Build history of the part. All positions in model axes, mm. A direction names the side the tool comes from. Round coordinates to 2 decimals unless told otherwise and drop trailing zeros. Loops run counter-clockwise (first coordinate to the right, second up) from the corner with the lowest first, then second, coordinate; pieces in that order, holes last. Notation, with made-up numbers: (76, -13) - (87, -13) arc R22 ccw to (87, -2) - close; hole circle Ø9 at (45.5, 45). An arc over 180 degrees is marked (long way). Put each result on its own line as item: value. Start each with the question number.
Autodesk Inventor part; units mm, degrees
ref_plane "РабПлоскость1" through (0, 28, 0) normal (0, 1, 0) x (-1, 0, 0)
ref_plane "YZ Plane" through (0, 0, 0) normal (1, 0, 0) x (0, 1, 0)
ref_plane "XY Plane" through (0, 0, 0) normal (0, 0, 1) x (1, 0, 0)
sketch "Эскиз1" plane through (0, 0, 0) normal (0, 1, 0) x (-1, 0, 0)
  line L0 (-2, 80) -> (2, 80)
  line L1 (2, 80) -> (2, -80)
  line L2 (2, -80) -> (-2, -80)
  line L3 (-2, -80) -> (-2, 80)
  line L4 (60, 32) -> (-60, 32)
  line L5 (-60, 32) -> (-60, 36)
  line L6 (-60, 36) -> (60, 36)
  line L7 (60, 36) -> (60, 32)
  line L8 (60, -32) -> (-60, -32)
  line L9 (-60, -32) -> (-60, -36)
  line L10 (-60, -36) -> (60, -36)
  line L11 (60, -36) -> (60, -32)
  line L12 (60, 32) -> (60, -32) construction
  line L13 (2, -80) -> (2, -80)
  line L14 (2, -80) -> (-2, -80)
  point P0 (0, 0)
  point P1 (0, -32)
  point P2 (60, 0)
  point P3 (0, -80)
  point P4 (2, 0)
  dimension "d1" = 120
  dimension "d3" = 4
  dimension "d4" = 4
  dimension "d5" = 4
  dimension "d26" = 32
  dimension "d27" = 32
  dimension "d28" = 80
  dimension "d29" = 80
  dimension "d32" = 44
extrude "Выдавливание1" add sketch "Эскиз1" along normal blind 56
ref_plane "РабПлоскость1" through (0, 28, 0) normal (0, 1, 0) x (-1, 0, 0)
sketch "Эскиз2" plane through (0, 0, 0) normal (0, 1, 0) x (-1, 0, 0)
  line L0 (-2, 36) -> (-2, 80) construction
  line L1 (-2, 80) -> (2, 80) construction
  line L2 (2, 80) -> (2, 36) construction
  line L3 (2, 36) -> (60, 36) construction
  line L4 (60, 36) -> (60, 32) construction
  line L5 (60, 32) -> (2, 32) construction
  line L6 (2, 32) -> (2, -32) construction
  line L7 (60, -32) -> (2, -32) construction
  line L8 (60, -36) -> (60, -32) construction
  line L9 (2, -36) -> (60, -36) construction
  line L10 (2, -36) -> (2, -80) construction
  line L11 (2, -80) -> (-2, -80) construction
  line L12 (-2, -80) -> (-2, -36) construction
  line L13 (-60, -36) -> (-2, -36) construction
  line L14 (-60, -32) -> (-60, -36) construction
  line L15 (-2, -32) -> (-60, -32) construction
  line L16 (-2, -32) -> (-2, 32) construction
  line L17 (-2, 32) -> (-60, 32) construction
  line L18 (-60, 32) -> (-60, 36) construction
  line L19 (-60, 36) -> (-2, 36) construction
  line L20 (-2, 32) -> (-6, 32)
  line L21 (-6, 32) -> (-6, 29)
  line L22 (-5, 28) -> (-2, 28)
  line L23 (-2, 28) -> (-2, 32)
  circle A0 centre (-4, 30) radius 1
  arc A1 (-6, 29) -> (-5, 28) centre (-5, 29) ccw
  line L24 (-2, -36) -> (-6, -36)
  line L25 (-6, -36) -> (-6, -39)
  line L26 (-5, -40) -> (-2, -40)
  line L27 (-2, -40) -> (-2, -36)
  circle A2 centre (-4, -38) radius 1
  arc A3 (-6, -39) -> (-5, -40) centre (-5, -39) ccw
  line L28 (-60, 34) -> (60, 34) construction
  line L29 (-60, -34) -> (60, -34) construction
  line L30 (0, 80) -> (0, -80) construction
  line L31 (-2, 36) -> (-6, 36)
  line L32 (-6, 36) -> (-6, 39)
  line L33 (-5, 40) -> (-2, 40)
  line L34 (-2, 40) -> (-2, 36)
  circle A4 centre (-4, 38) radius 1
  arc A5 (-5, 40) -> (-6, 39) centre (-5, 39) ccw
  line L35 (2, 32) -> (6, 32)
  line L36 (6, 32) -> (6, 29)
  line L37 (5, 28) -> (2, 28)
  line L38 (2, 28) -> (2, 32)
  circle A6 centre (4, 30) radius 1
  arc A7 (5, 28) -> (6, 29) centre (5, 29) ccw
  arc A8 (6, 39) -> (5, 40) centre (5, 39) ccw
  line L39 (5, 40) -> (2, 40)
  line L40 (2, 40) -> (2, 36)
  line L41 (6, 36) -> (6, 39)
  line L42 (2, 36) -> (6, 36)
  circle A9 centre (4, 38) radius 1
  line L43 (-2, -28) -> (-2, -32)
  line L44 (-2, -32) -> (-6, -32)
  circle A10 centre (-4, -30) radius 1
  line L45 (-6, -32) -> (-6, -29)
  arc A11 (-5, -28) -> (-6, -29) centre (-5, -29) ccw
  line L46 (-5, -28) -> (-2, -28)
  line L47 (2, -40) -> (2, -36)
  line L48 (2, -36) -> (6, -36)
  circle A12 centre (4, -38) radius 1
  line L49 (6, -36) -> (6, -39)
  arc A13 (5, -40) -> (6, -39) centre (5, -39) ccw
  line L50 (5, -40) -> (2, -40)
  line L51 (2, -28) -> (2, -32)
  line L52 (2, -32) -> (6, -32)
  line L53 (6, -32) -> (6, -29)
  line L54 (5, -28) -> (2, -28)
  arc A14 (6, -29) -> (5, -28) centre (5, -29) ccw
  circle A15 centre (4, -30) radius 1
  point P0 (0, 0)
  point P1 (-6, 28)
  point P2 (-6, -40)
  point P3 (-6, 40)
  point P4 (6, 28)
  point P5 (6, 40)
  point P6 (-6, -28)
  point P7 (2, -32)
  point P8 (6, -40)
  point P9 (6, -28)
  dimension "d11" = 4
  dimension "d12" = 4
  dimension "d13" = 2
  dimension "d15" = 1
  dimension "d16" = 2
  dimension "d17" = 2
  dimension "d18" = 4
  dimension "d19" = 4
  dimension "d20" = 2
  dimension "d21" = 1
  dimension "d22" = 2
  dimension "d23" = 2
extrude "Выдавливание2" add sketch "Эскиз2" along normal blind 2
mirror "Зеркальное отражение1" about plane through (0, 28, 0) normal (0, 1, 0) of "Выдавливание2"
extrude "Выдавливание3" add sketch "Эскиз1" along normal up to surface (56 mm away) contours L0 L1 L6 L3 | L6 L1 L4 L3 | L4 L1 L8 L3 | L8 L1 L10 L3 | L10 L1 L2 L3
properties part number "крепление-стенки" material "Пластик АБС"
1) Pull direction Y, two halves, no side cores. Call faces 1 (the face through (0, 0, 0)), 2 (the face through (-60, 28, 34)), 3 (the face through (-3, 2, -31)): pulls with the +Y half, pulls with the -Y half, needs draft (parallel to the pull), parting line crosses it, or undercut.
2) Which spindle directions (+Z, -Z, +X, -X, +Y, -Y) get a long thin tool onto all of the face, cutting with end or side? Do faces 4 (the face through (5, 2, -37)), 5 (the face through (3, 54, -31)), 6 (the face through (-3, 2, 39)). Say none if no direction does.
3) Slice it at C-C, the plane z = -43. Write the cut outline in (x, y).
4) Drop flat-ended pins along their axis: pin 1 Ø2 at (x, z) = (-4, 37.5) entering from -Y; pin 2 Ø6 at (x, y) = (37.5, 31.5) entering from -Z; pin 3 Ø8 at (y, z) = (25.5, -3) entering from +X; pin 4 Ø17 at (x, y) = (-30.5, 26.5) entering from +Z. Give the stop position or say it passes through.
5) Slice it at B-B, the plane y = 47.5. Write the cut outline in (x, z), and give its area (3 significant figures).
6) Drill centre lines: line 1 (Z direction, x = 4, y = 55); line 2 (Z direction, x = -25, y = 21.5); line 3 (X direction, y = 35.5, z = -20). Where is each one in solid material? Low to high. Write a range as [from, to].
7) Slice it at A-A, the plane x = 50.5. Write the cut outline in (y, z).
Taken from the geometry:
1. face 1: pulls with the -Y half
1. face 2: needs draft
1. face 3: undercut
2. face 4: -Z, +X
2. face 5: +X
2. face 6: +Z, -X
3. outline: (-2, 0) - (2, 0) - (2, 56) - (-2, 56) - close
4. pin 1: stops at y = 0
4. pin 2: stops at z = -36
4. pin 3: stops at x = 2
4. pin 4: stops at z = 36
5. outline: (-60, -36) - (-2, -36) - (-2, -80) - (2, -80) - (2, -36) - (60, -36) - (60, -32) - (2, -32) - (2, 32) - (60, 32) - (60, 36) - (2, 36) - (2, 80) - (-2, 80) - (-2, 36) - (-60, 36) - (-60, 32) - (-2, 32) - (-2, -32) - (-60, -32) - close
5. area: 1,570 mm2
6. line 1: z = [-40, -39], [-37, -31], [-29, -28], [28, 29], [31, 37], [39, 40]
6. line 2: z = [-36, -32], [32, 36]
6. line 3: x = [-2, 2]
7. outline: (0, -36) - (56, -36) - (56, -32) - (0, -32) - close; (0, 32) - (56, 32) - (56, 36) - (0, 36) - close
